Read the model definition and answer for the solid it produces. Units are mm, in the model's axes. A direction names the side the tool comes from. Round coordinates to 2 decimals unless told otherwise and drop trailing zeros. Loops run counter-clockwise (first coordinate to the right, second up) from the corner with the lowest first, then second, coordinate; pieces in that order, holes last. Notation, with made-up numbers: (80, 54.25) - (99, 54.25) arc R24 cw to (99, 83.25) - close; hole circle Ø1 at (81, 66). An arc over 180 degrees is marked (long way). Answer as CSV lines item,"result".
```python
from build123d import *

# Parameters (mm, degrees)
SKETCH_W        = 165
SKETCH_H        = 105
PAD_DEPTH       = 27
SKETCH001_W     = 158
SKETCH001_H     = 98
POCKET_DEPTH    = 25
SKETCH002_W     = 161.5
SKETCH002_H     = 101.5
POCKET001_DEPTH = 12
SKETCH003_R     = 10
POCKET002_DEPTH = 27.001
SKETCH004_W     = 17.5
SKETCH004_H     = 9
POCKET003_DEPTH = 24.5
SKETCH005_W     = 15
SKETCH005_H     = 8
POCKET004_DEPTH = 20.5


with BuildPart() as part:
    # Sketch → Pad (new body)
    with BuildSketch(Plane.XY):
        with Locations((82.5, 52.5)):
            Rectangle(SKETCH_W, SKETCH_H)
    extrude(amount=PAD_DEPTH)

    # Sketch001 → Pocket (cut)
    with BuildSketch(Plane.XY.offset(27)):
        with Locations((82.5, 52.5)):
            Rectangle(SKETCH001_W, SKETCH001_H)
    extrude(amount=-POCKET_DEPTH, mode=Mode.SUBTRACT)

    # Sketch002 → Pocket001 (cut)
    with BuildSketch(Plane.XY.offset(27)):
        with Locations((82.5, 52.5)):
            Rectangle(SKETCH002_W, SKETCH002_H)
    extrude(amount=-POCKET001_DEPTH, mode=Mode.SUBTRACT)

    # Sketch003 → Pocket002 (cut, through all)
    with BuildSketch(Plane(origin=(0, 0, 0), x_dir=(1, 0, 0), z_dir=(0, 0, -1))):
        with Locations((15, -85.5)):
            Circle(SKETCH003_R)
        with Locations((38, -85.5)):
            Circle(SKETCH003_R)
        with Locations((71, -85.5)):
            Circle(SKETCH003_R)
        with Locations((94, -85.5)):
            Circle(SKETCH003_R)
        with Locations((127, -85.5)):
            Circle(SKETCH003_R)
        with Locations((150, -85.5)):
            Circle(SKETCH003_R)
    extrude(amount=-POCKET002_DEPTH, mode=Mode.SUBTRACT)

    # Sketch004 → Pocket003 (cut)
    with BuildSketch(Plane.XY.offset(27)):
        with Locations((156.25, 7)):
            Rectangle(SKETCH004_W, SKETCH004_H)
    extrude(amount=-POCKET003_DEPTH, mode=Mode.SUBTRACT)

    # Sketch005 → Pocket004 (cut)
    with BuildSketch(Plane.XY.offset(27)):
        with Locations((157.5, 21)):
            Rectangle(SKETCH005_W, SKETCH005_H)
    extrude(amount=-POCKET004_DEPTH, mode=Mode.SUBTRACT)


solid = part.part
```
1) Find the intervals of material crossed by line 1 (Y direction, x = 75, z = 20.25); line 2 (Y direction, x = 71, z = 0.5); line 3 (X direction, y = 55.5, z = 21.5), in increasing order.
Entries:
line 1,"y = 0 to 1.75, 103.25 to 105"
line 2,"y = 0 to 75.5, 95.5 to 105"
line 3,"x = 0 to 1.75, 163.25 to 165"
2) A cutting plane is placed at C-C, the plane y = 85.5. Count the separate pieces of the cut face and the enclosed holes in it, plus the area to 3 significant figures.
Entries:
separate pieces,"7"
enclosed holes,"0"
area,"223 mm^2"
3) The mould has two halves that part along Y. Classify faces 1 (the face through (81, 53, 0)), 2 (the face through (3.5, 52, 9)), 3 (the face through (81, 105, 13)): pulls with the +Y half, pulls with the -Y half, needs draft (parallel to the pull), parting line crosses it, or undercut.
Entries:
face 1,"needs draft"
face 2,"undercut"
face 3,"pulls with the +Y half"
4) A cutting plane is placed at D-D, the plane x = 150. Determine the outline of the cut face in (y, z).
Entries:
outline,"(0, 0) - (75.5, 0) - (75.5, 2) - (3.5, 2) - (3.5, 2.5) - (2.5, 2.5) - (2.5, 15) - (1.75, 15) - (1.75, 27) - (0, 27) - close; (95.5, 0) - (105, 0) - (105, 27) - (103.25, 27) - (103.25, 15) - (101.5, 15) - (101.5, 2) - (95.5, 2) - close"
5) This flat-tipped pin is pushed along its axis until it touches: P1, Ø1, axis at x = 162.5, y = 21.5, coming from the +Z side. Where does it stop, or does it pass through?
Entries:
P1,"stops at z = 6.5"
6) A cutting plane is placed at A-A, the plane z = 12. Determine the outline of the cut face in (x, y).
Entries:
outline,"(0, 0) - (165, 0) - (165, 2.5) - (147.5, 2.5) - (147.5, 3.5) - (3.5, 3.5) - (3.5, 101.5) - (161.5, 101.5) - (161.5, 25) - (165, 25) - (165, 105) - (0, 105) - close; (161.5, 11.5) - (165, 11.5) - (165, 17) - (161.5, 17) - close"
7) A tool of negligible diameter and unlimited length cuts with its end or side. For faces 4 (the face through (81, 101.5, 9)), 5 (the face through (0, 52, 13)), 6 (the face through (163, 21, 6.5)), from which of +Z, -Z, +X, -X, +Y, -Y can it reach the whole face along a straight path? Write none if from no direction.
Entries:
face 4,"+Z"
face 5,"+Z, -Z, -X, +Y, -Y"
face 6,"+Z, +X"
8) A cutting plane is placed at B-B, the plane x = 102. Determine the outline of the cut face in (y, z).
Entries:
outline,"(0, 0) - (79.5, 0) - (79.5, 2) - (3.5, 2) - (3.5, 15) - (1.75, 15) - (1.75, 27) - (0, 27) - close; (91.5, 0) - (105, 0) - (105, 27) - (103.25, 27) - (103.25, 15) - (101.5, 15) - (101.5, 2) - (91.5, 2) - close"
